CAD build for the part. Positions are in the model's coordinates, mm. A direction names the side the tool comes from. Give positions to 0.01 mm unless a question says otherwise; leave off trailing zeros. Write each loop counter-clockwise with the first axis right and the second up, starting at its lowest first coordinate (ties: lowest second). Pieces come first, ordered by that corner, then holes. Notation, with made-up numbers: M 12.5,16.5 L 48.5,16.5 A15 ccw 48.5,39.5 Z; hole C -23.75,-19.5 d10. An arc over 180 degrees is marked long. One line per question, with ' | ' between items. Start each with the question number.
1. Flat gauge pins, fed straight in: pin 1 (1.4 mm diameter, centred on x = 2.5, y = 12.5, fed in from +Z); pin 2 (0.9 mm diameter, centred on y = 1.5, z = 10.5, fed in from +X); pin 3 (4.5 mm diameter, centred on x = 7, y = 0.5, fed in from -Z). Where does each tip first touch, or does it go through?
2. Cut at D-D, the plane z = 10. Write the cut outline in (x, y) (3 decimals), then the cut area to 3 significant figures.
3. Cut at B-B, the plane y = -12.5. Write the cut outline in (x, z), then the cut area to 3 significant figures.
4. Wall check: L1, parallel to Y at x = 27.5, z = 9; L2, parallel to Y at x = 2.5, z = 12; L3, parallel to Y at x = 21.45, z = 14.2. Give the ranges that are in metal, low to high.
5. Which spindle directions (+Z, -Z, +X, -X, +Y, -Y) get a long thin tool onto all of the face, cutting with end or side? Do faces 1 (the face through (22.3, -2.1, 12)), 2 (the face through (8.523, 1.774, 8.797)), 3 (the face through (24.1, 0.06, 13.52)). Say none if no direction does.
6. Cut at C-C, the plane x = 2.5. Write the cut outline in (y, z).
7. Cut at A-A, the plane z = 6.5. Write the cut outline in (x, y).
8. Pull direction X, two halves, no side cores. Call faces 4 (the face through (14.07, 5.73, 13.52)), 5 (the face through (8, 7, 18)), 6 (the face through (10.892, 9.007, 10.479)): released by +X, released by -X, zero draft, split by the parting line, or undercut.
```python
from build123d import *

# Parameters (mm, degrees)
SKETCH2_W              = 30
SKETCH2_H              = 30
SKETCH2_R              = 5
SKETCH2_R_2            = 1.025
BOSS_EXTRUDE1_DEPTH    = 18
SKETCH3_W              = 30
SKETCH3_H              = 20
CUT_EXTRUDE1_DEPTH     = 9
F_2_56_TAPPED_HOLE1_D  = 1.778
CUT_EXTRUDE2_START     = -3
SKETCH8_R              = 10.1
SKETCH8_R_2            = 5
SKETCH8_R_3            = 1.025
CUT_EXTRUDE2_DEPTH     = 3
BOSS_EXTRUDE2_START    = 0.4
SKETCH9_R              = 2
SKETCH9_R_2            = 1.025
BOSS_EXTRUDE2_DEPTH    = 0.4
SKETCH10_W             = 20.050000056
SKETCH10_H             = 20
CUT_EXTRUDE3_DEPTH     = 2.999999892
FILLET1_START          = 9
FILLET1_DEPTH          = 4
M2_5_CLEARANCE_HOLE1_D = 2.7


with BuildPart() as part:
    # Sketch2 → Boss-Extrude1 (new body)
    # profile 1 of 2: a face of its own
    with BuildSketch(Plane.XY):
        with Locations((15, 0)):
            Rectangle(SKETCH2_W, SKETCH2_H)
        with Locations((17.449999944, 0)):
            Circle(SKETCH2_R, mode=Mode.SUBTRACT)
        with Locations((7.599999986, 0)):
            Circle(SKETCH2_R_2, mode=Mode.SUBTRACT)
    # profile 2 of 2: a face of its own
    with BuildSketch(Plane.XY):
        with BuildLine():
            ThreePointArc((22.449999944, 0), (20.98553385, -3.535533906), (17.449999944, -5))
            Line((17.449999944, -5), (30, -5))
            Line((30, -5), (30, 5))
            Line((30, 5), (17.449999944, 5))
            ThreePointArc((17.449999944, 5), (20.98553385, 3.535533906), (22.449999944, 0))
        make_face()
    extrude(amount=BOSS_EXTRUDE1_DEPTH)

    # Sketch3 → Cut-Extrude1 (cut)
    with BuildSketch(Plane(origin=(0, 0, 0), x_dir=(-1, 0, 0), z_dir=(0, 0, -1))):
        with Locations((-15, 0)):
            Rectangle(SKETCH3_W, SKETCH3_H)
    extrude(amount=-CUT_EXTRUDE1_DEPTH, mode=Mode.SUBTRACT)

    # #2-56 Tapped Hole1 (through all)
    with Locations(Plane(origin=(0, 0, 0), x_dir=(-1, 0, 0), z_dir=(0, 0, -1))):
        with Locations((-27.5, 12.5), (-27.5, -12.5), (-2.5, -12.5), (-2.5, 12.5)):
            Hole(F_2_56_TAPPED_HOLE1_D / 2)

    # Sketch8 → Cut-Extrude2 (cut)
    # profile 1 of 2: a face of its own
    with BuildSketch(Plane.XY.offset(18).offset(CUT_EXTRUDE2_START)):
        with Locations((17.449999944, 0)):
            Circle(SKETCH8_R)
        with Locations(Location((17.449999944, 0, 0), (0, 0, 180))):
            Circle(SKETCH8_R_2, mode=Mode.SUBTRACT)
    # profile 2 of 2: a face of its own
    with BuildSketch(Plane.XY.offset(18).offset(CUT_EXTRUDE2_START)):
        with Locations(Location((7.599999986, 0, 0), (0, 0, 180))):
            Circle(SKETCH8_R_3)
    extrude(amount=CUT_EXTRUDE2_DEPTH, mode=Mode.SUBTRACT)

    # Sketch9 → Boss-Extrude2 (add)
    with BuildSketch(Plane(origin=(0, 0, 9), x_dir=(-1, 0, 0), z_dir=(0, 0, -1)).offset(BOSS_EXTRUDE2_START)):
        with Locations(Location((-7.599999986, 0, 0), (0, 0, 180))):
            Circle(SKETCH9_R)
        with Locations(Location((-7.599999986, 0, 0), (0, 0, 78.757190581))):
            Circle(SKETCH9_R_2, mode=Mode.SUBTRACT)
    extrude(amount=-BOSS_EXTRUDE2_DEPTH)

    # Sketch10 → Cut-Extrude3 (cut)
    with BuildSketch(Plane(origin=(0, 0, 9), x_dir=(-1, 0, 0), z_dir=(0, 0, -1))):
        with Locations((-19.974999972, 0)):
            Rectangle(SKETCH10_W, SKETCH10_H)
    extrude(amount=-CUT_EXTRUDE3_DEPTH, mode=Mode.SUBTRACT)

    # Fillet1: read off the stored shape, not the designer's step
    # Fillet1 outline → Fillet1 (add)
    with BuildSketch(Plane.XY.offset(FILLET1_START)):
        with BuildLine():
            Line((9.949999944, -10), (13.251999944, -10))
            ThreePointArc((13.251999944, -10), (10.917133353, -9.032866591), (9.949999944, -6.698))
            Line((9.949999944, -6.698), (9.949999944, -10))
        make_face()
        with BuildLine():
            Line((9.949999944, 10), (9.949999944, 6.698))
            ThreePointArc((9.949999944, 6.698), (10.917133353, 9.032866591), (13.251999944, 10))
            Line((13.251999944, 10), (9.949999944, 10))
        make_face()
    extrude(amount=FILLET1_DEPTH)

    # M2.5 Clearance Hole1 (through all)
    with Locations(Plane(origin=(0, 0, 11.999999892), x_dir=(-1, 0, 0), z_dir=(0, 0, -1))):
        with Locations((-21.449999944, 6.92820323), (-13.449999944, 6.92820323), (-13.285717643, -7.212748522), (-21.449999944, -6.92820323), (-25.449999944, 0)):
            Hole(M2_5_CLEARANCE_HOLE1_D / 2)


solid = part.part
```
Here are the results:
1) pin 1: through | pin 2: x = 9.95 | pin 3: z = 8.6
2) outline: M 0,-15 L 30,-15 L 30,-10 L 13.252,-10 A3.302 cw 9.95,-6.698 L 9.95,6.698 A3.302 cw 13.252,10 L 30,10 L 30,15 L 0,15 Z; hole C 2.5,-12.5 d1.778; hole C 2.5,12.5 d1.778; hole C 7.6,0 d2.05; hole C 27.5,-12.5 d1.778; hole C 27.5,12.5 d1.778 | area: 490 mm^2
3) outline: M 0,0 L 1.61,0 L 1.61,18 L 0,18 Z; M 3.39,0 L 26.61,0 L 26.61,18 L 3.39,18 Z; M 28.39,0 L 30,0 L 30,18 L 28.39,18 Z | area: 476 mm^2
4) L1: -15 to -13.39, -11.61 to -10, 10 to 11.61, 13.39 to 15 | L2: -15 to -13.39, -11.61 to 11.61, 13.39 to 15 | L3: -15 to -8.28, -5.58 to -3, 3 to 5.58, 8.28 to 15
5) face 1: -Z, +X | face 2: -Z | face 3: +Z, -Z
6) outline: M -15,0 L -13.39,0 L -13.39,18 L -15,18 Z; M -11.61,0 L -10,0 L -10,9 L 10,9 L 10,0 L 11.61,0 L 11.61,18 L -11.61,18 Z; M 13.39,0 L 15,0 L 15,18 L 13.39,18 Z
7) outline: M 0,-15 L 30,-15 L 30,-10 L 0,-10 Z; M 0,10 L 30,10 L 30,15 L 0,15 Z; hole C 2.5,-12.5 d1.78; hole C 2.5,12.5 d1.78; hole C 27.5,-12.5 d1.78; hole C 27.5,12.5 d1.78
8) face 4: undercut | face 5: zero draft | face 6: released by +X
